```python
from build123d import *

# Parameters (mm, degrees)
F0_W     = 762
F0_H     = 609.6
F1_DEPTH = 2286
F2_W     = 762
F2_H     = 101.6
F3_DEPTH = 76.2
F4_W     = 279.4
F4_H     = 990.6
F4_W_2   = 1.27
F4_H_2   = 2184.4
F5_DEPTH = 25.4


with BuildPart() as f1:
    # F0 (on Top) → F1 (new body)
    with BuildSketch(Plane.XY):
        with Locations((76.2, 0)):
            Rectangle(F0_W, F0_H)
    extrude(amount=F1_DEPTH)

    # F2 (on face) → F3 (cut)
    with BuildSketch(Plane.XZ.offset(304.8)):
        with Locations((76.2, 50.8)):
            Rectangle(F2_W, F2_H)
    extrude(amount=-F3_DEPTH, mode=Mode.SUBTRACT)

    # F4 (on face) → F5 (cut)
    with BuildSketch(Plane.XZ.offset(304.8)):
        with Locations((-114.3, 1739.9)):
            Rectangle(F4_W, F4_H)
        with Locations((266.7, 1739.9)):
            Rectangle(F4_W, F4_H)
        with Locations((266.7, 647.7)):
            Rectangle(F4_W, F4_H)
        with Locations((-114.3, 647.7)):
            Rectangle(F4_W, F4_H)
        with Locations((76.2, 1193.8)):
            Rectangle(F4_W_2, F4_H_2)
    extrude(amount=-F5_DEPTH, mode=Mode.SUBTRACT)


solid = f1.part
```
Can you work these out from the model? Positions are in its coordinate system, mm. A direction names the side the tool comes from. Coordinates: 2 decimals unless noted, no trailing zeros. Loops run counter-clockwise (first coordinate to the right, second up) from the corner with the lowest first, then second, coordinate; pieces in that order, holes last.
Item 1: Please list where these lines run through material, in increasing order: L1, parallel to Y at x = 305, z = 511; L2, parallel to Z at x = 41, y = -248.
Answers below:
L1: y = -279.4 to 304.8
L2: z = 101.6 to 2286
Item 2: Suppose I cut it at A-A (z = 576). Please give me the cut outline in (x, y) (3 decimals).
Answers below:
outline: (-304.8, -304.8) - (-254, -304.8) - (-254, -279.4) - (25.4, -279.4) - (25.4, -304.8) - (75.565, -304.8) - (75.565, -279.4) - (76.835, -279.4) - (76.835, -304.8) - (127, -304.8) - (127, -279.4) - (406.4, -279.4) - (406.4, -304.8) - (457.2, -304.8) - (457.2, 304.8) - (-304.8, 304.8) - close
Item 3: If we mould it in two halves opening along X, with no side actions, what happens to faces 4 (the face through (-304.8, -4, 1127)), 5 (the face through (71, -267, 101.6)), 6 (the face through (-116, -279.4, 655))? For each: released by +X, released by -X, zero draft, split by the parting line, or undercut.
Answers below:
face 4: released by -X
face 5: zero draft
face 6: undercut
Item 4: I'm going to push a flat-ended pin straight in: pin 1 (20.5 mm diameter, centred on x = 238, y = -294, fed in from -Z). Where does the tip first touch, or does it pass through?
Answers below:
pin 1: stops at z = 101.6
Item 5: Which directions (+Z, -Z, +X, -X, +Y, -Y) give clear straight access to the entire face, cutting with the end or side of a thin tool? Please do faces 1 (the face through (71, -228.6, 52)), 2 (the face through (457.2, -4, 1127)), 3 (the face through (265, -279.4, 1747)).
Answers below:
face 1: -Z, +X, -X, -Y
face 2: +Z, -Z, +X, +Y, -Y
face 3: -Y
Item 6: Suppose I cut it at B-B (x = 305). Please give me the cut outline in (y, z), then the cut area to 3 significant figures.
Answers below:
outline: (-304.8, 101.6) - (-228.6, 101.6) - (-228.6, 0) - (304.8, 0) - (304.8, 2286) - (-304.8, 2286) - (-304.8, 2235.2) - (-279.4, 2235.2) - (-279.4, 1244.6) - (-304.8, 1244.6) - (-304.8, 1143) - (-279.4, 1143) - (-279.4, 152.4) - (-304.8, 152.4) - close
area: 1,340,000 mm2
